Could you check a few things on this model? Use its own coordinates, in mm. Give positions to 0.01 mm unless a question says otherwise; leave off trailing zeros. Write each loop counter-clockwise with the first axis right and the second up, starting at its lowest first coordinate (ties: lowest second). Pieces come first, ordered by that corner, then holes. Notation, with made-up numbers: (-7.5, 10.25) - (-2.5, 10.25) arc R26 cw to (-2.5, 40.25) - close; hole circle Ø3 at (-22.5, 12). An arc over 180 degrees is marked (long way). Use one line per item in the form item = value.
```python
from build123d import *

# Parameters (mm, degrees)
SKETCH1_R           = 1.65
BOSS_EXTRUDE1_DEPTH = 12.7


with BuildPart() as part:
    # Sketch1 → Boss-Extrude1 (new body)
    with BuildSketch(Plane(origin=(0, 0, 0), x_dir=(1, 0, 0), z_dir=(0, 1, 0))):
        with BuildLine():
            ThreePointArc((-111.234035703, -19.613561667), (-112.95, 0), (-111.234035703, 19.613561667))
            ThreePointArc((-111.234035703, 19.613561667), (-109.13025705, 22.87401705), (-105.327953741, 23.647931427))
            ThreePointArc((-105.327953741, 23.647931427), (0, 107.95), (105.327953741, 23.647931427))
            ThreePointArc((105.327953741, 23.647931427), (109.13025705, 22.87401705), (111.234035703, 19.613561667))
            ThreePointArc((111.234035703, 19.613561667), (112.95, 0), (111.234035703, -19.613561667))
            ThreePointArc((111.234035703, -19.613561667), (109.13025705, -22.87401705), (105.327953741, -23.647931427))
            ThreePointArc((105.327953741, -23.647931427), (0, -107.95), (-105.327953741, -23.647931427))
            ThreePointArc((-105.327953741, -23.647931427), (-109.13025705, -22.87401705), (-111.234035703, -19.613561667))
        make_face()
        with Locations(Location((0, 104.55, 0), (0, 0, 270))):
            Circle(SKETCH1_R, mode=Mode.SUBTRACT)
        with Locations(Location((52.275, 90.542955966, 0), (0, 0, 270))):
            Circle(SKETCH1_R, mode=Mode.SUBTRACT)
        with Locations(Location((90.542955966, 52.275, 0), (0, 0, 270))):
            Circle(SKETCH1_R, mode=Mode.SUBTRACT)
        with Locations(Location((104.55, 0, 0), (0, 0, 270))):
            Circle(SKETCH1_R, mode=Mode.SUBTRACT)
        with Locations(Location((90.542955966, -52.275, 0), (0, 0, 270))):
            Circle(SKETCH1_R, mode=Mode.SUBTRACT)
        with Locations(Location((52.275, -90.542955966, 0), (0, 0, 270))):
            Circle(SKETCH1_R, mode=Mode.SUBTRACT)
        with Locations(Location((0, -104.55, 0), (0, 0, 270))):
            Circle(SKETCH1_R, mode=Mode.SUBTRACT)
        with Locations(Location((-52.275, -90.542955966, 0), (0, 0, 270))):
            Circle(SKETCH1_R, mode=Mode.SUBTRACT)
        with Locations(Location((-90.542955966, -52.275, 0), (0, 0, 270))):
            Circle(SKETCH1_R, mode=Mode.SUBTRACT)
        with Locations(Location((-104.55, 0, 0), (0, 0, 270))):
            Circle(SKETCH1_R, mode=Mode.SUBTRACT)
        with Locations(Location((-90.542955966, 52.275, 0), (0, 0, 270))):
            Circle(SKETCH1_R, mode=Mode.SUBTRACT)
        with Locations(Location((-52.275, 90.542955966, 0), (0, 0, 270))):
            Circle(SKETCH1_R, mode=Mode.SUBTRACT)
    extrude(amount=BOSS_EXTRUDE1_DEPTH)


solid = part.part
```
1. Imagine slicing it at C-C, the plane z = -66. List the corners of the cut face in (x, y) for me.
Response values:
outline = (-85.42, 0) - (85.42, 0) - (85.42, 12.7) - (-85.42, 12.7) - close
2. Imagine slicing it at B-B, the plane x = -58.5. List the corners of the cut face in (y, z) for me, and give its area (3 significant figures).
Response values:
outline = (0, -90.72) - (12.7, -90.72) - (12.7, 90.72) - (0, 90.72) - close
area = 2,300 mm²
3. Imagine slicing it at A-A, the plane y = 2.5. State how many separate pieces and enclosed holes the cut face has, and give its area (3 significant figures).
Response values:
separate_pieces = 1
enclosed_holes = 12
area = 37,000 mm²
4. For pin 1 (5 mm diameter, centred on y = 4.5, z = -59.5, fed in from +X); pin 2 (5 mm diameter, centred on y = 9, z = -59.5, fed in from -X); pin 3 (6 mm diameter, centred on y = 3.5, z = -61, fed in from -X), each with a flat end and sliding along its axis, tell me the tip position at first contact or that it passes through.
Response values:
pin_1 = 91.67
pin_2 = -91.67
pin_3 = -91.05
5. If I drill on line 1 (X direction, y = 8.5, z = 77.5); line 2 (X direction, y = 7.5, z = 28.5); line 3 (Z direction, x = 65.5, y = 0.5), over which ranges is the centre line in solid material (lowest first)? Write a range as from..to.
Response values:
line_1 = -75.15..75.15
line_2 = -104.12..104.12
line_3 = -85.81..85.81
